Autodesk Inventor part; units mm, degrees
ref_plane "YZ Plane" through (0, 0, 0) normal (1, 0, 0) x (0, 1, 0)
ref_plane "XZ Plane" through (0, 0, 0) normal (0, 1, 0) x (-1, 0, 0)
ref_plane "XY Plane" through (0, 0, 0) normal (0, 0, 1) x (1, 0, 0)
sketch "Boceto1" plane through (0, 0, 0) normal (0, 1, 0) x (-1, 0, 0)
  line L0 (-75, -125) -> (75, -125)
  line L1 (75, -125) -> (75, 125)
  line L2 (75, 125) -> (-75, 125)
  line L3 (-75, 125) -> (-75, -125)
  line L4 (-75, -125) -> (75, 125) construction
  line L5 (75, -125) -> (-75, 125) construction
  line L6 (70, 120) -> (70, -120)
  line L7 (70, -120) -> (-70, -120)
  line L8 (-70, -120) -> (-70, 120)
  line L9 (-70, 120) -> (70, 120)
  line L10 (-75, 125) -> (-75, 100)
  line L11 (-75, 100) -> (-70, 100) construction
  line L12 (-75, 100) -> (-75, 50)
  line L13 (-75, 50) -> (-70, 50) construction
  line L14 (-75, 50) -> (-75, 0)
  line L15 (-75, 100.5) -> (-70, 100.5)
  line L16 (-70, 100.5) -> (-70, 99.5)
  line L17 (-70, 99.5) -> (-75, 99.5)
  line L18 (-75, 99.5) -> (-75, 100.5)
  line L19 (-75, 100.5) -> (-70, 99.5) construction
  line L20 (-70, 100.5) -> (-75, 99.5) construction
  line L21 (-75, 49.5) -> (-70, 49.5)
  line L22 (-70, 49.5) -> (-70, 50.5)
  line L23 (-70, 50.5) -> (-75, 50.5)
  line L24 (-75, 50.5) -> (-75, 49.5)
  line L25 (-75, 49.5) -> (-70, 50.5) construction
  line L26 (-70, 49.5) -> (-75, 50.5) construction
  line L27 (0, 125) -> (-20, 125) construction
  line L28 (-20, 125) -> (-40, 125) construction
  line L29 (-40, 125) -> (-60, 125) construction
  line L30 (-20, 125) -> (-20, 120) construction
  line L31 (-40, 125) -> (-40, 120) construction
  line L32 (-60, 125) -> (-60, 120) construction
  line L33 (-20.5, 120) -> (-19.5, 120)
  line L34 (-19.5, 120) -> (-19.5, 125)
  line L35 (-19.5, 125) -> (-20.5, 125)
  line L36 (-20.5, 125) -> (-20.5, 120)
  line L37 (-20.5, 120) -> (-19.5, 125) construction
  line L38 (-19.5, 120) -> (-20.5, 125) construction
  line L39 (-40.5, 120) -> (-39.5, 120)
  line L40 (-39.5, 120) -> (-39.5, 125)
  line L41 (-39.5, 125) -> (-40.5, 125)
  line L42 (-40.5, 125) -> (-40.5, 120)
  line L43 (-40.5, 120) -> (-39.5, 125) construction
  line L44 (-39.5, 120) -> (-40.5, 125) construction
  line L45 (-60.5, 120) -> (-59.5, 120)
  line L46 (-59.5, 120) -> (-59.5, 125)
  line L47 (-59.5, 125) -> (-60.5, 125)
  line L48 (-60.5, 125) -> (-60.5, 120)
  line L49 (-60.5, 120) -> (-59.5, 125) construction
  line L50 (-59.5, 120) -> (-60.5, 125) construction
  line L51 (0, 125) -> (0, 120) construction
  line L52 (-0.5, 120) -> (0.5, 120)
  line L53 (0.5, 120) -> (0.5, 125)
  line L54 (0.5, 125) -> (-0.5, 125)
  line L55 (-0.5, 125) -> (-0.5, 120)
  line L56 (-0.5, 120) -> (0.5, 125) construction
  line L57 (0.5, 120) -> (-0.5, 125) construction
  line L58 (-70, 0) -> (-75, 0) construction
  line L59 (-75, -0.5) -> (-70, -0.5)
  line L60 (-70, -0.5) -> (-70, 0.5)
  line L61 (-70, 0.5) -> (-75, 0.5)
  line L62 (-75, 0.5) -> (-75, -0.5)
  line L63 (-75, -0.5) -> (-70, 0.5) construction
  line L64 (-70, -0.5) -> (-75, 0.5) construction
  point P0 (0, 0)
  point P1 (-72.5, 100)
  point P2 (-72.5, 50)
  point P3 (-20, 122.5)
  point P4 (-40, 122.5)
  point P5 (-60, 122.5)
  point P6 (0, 122.5)
  point P7 (-72.5, 0)
  point P8 (-75, 0.5)
  point P9 (-75, -0.5)
  point P10 (-70, -0.5)
  point P11 (-75, 50.5)
  point P12 (-75, 49.5)
  point P13 (-70, 100.5)
  point P14 (-0.5, 125)
  point P15 (-0.5, 120)
  point P16 (0.5, 120)
  point P17 (0.5, 125)
  point P18 (-20.5, 125)
  point P19 (-19.5, 125)
  point P20 (-40.5, 125)
  point P21 (-40.5, 120)
  point P22 (-39.5, 120)
  point P23 (-39.5, 125)
  point P24 (-60.5, 120)
  point P25 (-59.5, 120)
  point P26 (-59.5, 125)
  dimension "d0" = 150
  dimension "d1" = 250
  dimension "d2" = 5
  dimension "d5" = 25
  dimension "d6" = 50
  dimension "d7" = 50
  dimension "d8" = 1
  dimension "d9" = 1
  dimension "d10" = 20
  dimension "d11" = 20
  dimension "d12" = 20
  dimension "d13" = 1
  dimension "d14" = 1
  dimension "d15" = 1
  dimension "d16" = 1
  dimension "d17" = 1
extrude "Extrusión1" add sketch "Boceto1" along normal blind 3 contours L3 L59 L8 L7 L6 L9 L53 L2 L1 L0 | L3 L61 L8 L59 | L53 L9 L55 L2 | L3 L21 L8 L61 | L55 L9 L34 L2 | L3 L23 L8 L21 | L34 L9 L36 L2 | L23 L3 L17 L8 | L36 L9 L40 L2 | L17 L3 L15 L8 | L40 L9 L42 L2 | L15 L3 L2 L48 L9 L8 | L42 L9 L46 L2 | L46 L9 L48 L2
extrude "Extrusión2" add sketch "Boceto1" against normal blind 0.2 contours L3 L61 L8 L59 | L53 L9 L55 L2 | L3 L23 L8 L21 | L34 L9 L36 L2 | L17 L3 L15 L8 | L40 L9 L42 L2 | L46 L9 L48 L2
mirror "Simetría1" about plane through (0, 0, 0) normal (1, 0, 0) of "Extrusión2", "Extrusión1"
mirror "Simetría2" about plane through (0, 0, 0) normal (0, 0, 1) of "Extrusión2", "Extrusión1", "Simetría1"
ref_plane "Plano de trabajo1" through (0, 0, 0) normal (1, 0, 0) x (0, 1, 0)
ref_plane "Plano de trabajo2" through (0, 0, 0) normal (-1, 0, 0) x (0, 1, 0)
ref_plane "Plano de trabajo3" through (0, 0, 0) normal (-1, 0, 0) x (0, 1, 0)
properties part number "medidor"
Model file for the job. Use its own axes, mm. A direction names the side the tool comes from. Coordinates: 2 decimals unless noted, no trailing zeros. Loops run counter-clockwise (first coordinate to the right, second up) from the corner with the lowest first, then second, coordinate; pieces in that order, holes last. Notation, with made-up numbers: (67.5, 80.25) - (114.5, 80.25) arc R22 cw to (114.5, 95.25) - close; hole circle Ø5 at (-17.5, -3). An arc over 180 degrees is marked (long way). Write item = value, one per line. Start each with the question number.
Item 1: Saw through at B-B, the plane x = -7.5. List the corners of the cut face in (y, z), then the cut area to 3 significant figures.
Item 2: Saw through at C-C, the plane z = 63. List the corners of the cut face in (x, y), then the cut area to 3 significant figures.
Item 3: Wall check: probe 1 along X at (y, z) = (2.85, 106); probe 2 along Z at (x, y) = (7, 0.45). Give the ranges that are in metal, low to high. Write a range as [from, to].
Item 4: Saw through at A-A, the plane y = 0.6. List the corners of the cut face in (x, z), then the cut area to 3 significant figures.
Item 5: Drop a flat-ended pin along its axis: pin 1 Ø1.5 at (x, z) = (71.5, 64.5) entering from -Y. Give the stop position or say it passes through.
Item 6: 3-axis set-ups, long thin cutter, end or side, ignore diameter. For faces 3 (the face through (73, 0, -75)), 4 (the face through (10, 0, -122)), 5 (the face through (71, 0, 116)): which of +Z, -Z, +X, -X, +Y, -Y reach the whole face in a straight line?
Item 7: Pull direction Z, two halves, no side cores. Call faces 1 (the face through (-71, 0, 116)), 2 (the face through (-72, 0, -25)): +Z half, -Z half, draft (parallel to the pull), parting line (faces both ways), or undercut.
Answers:
q1.outline = (0, -125) - (3, -125) - (3, -120) - (0, -120) - close; (0, 120) - (3, 120) - (3, 125) - (0, 125) - close
q1.area = 30.0 mm2
q2.outline = (-75, 0) - (-70, 0) - (-70, 3) - (-75, 3) - close; (70, 0) - (75, 0) - (75, 3) - (70, 3) - close
q2.area = 30.0 mm2
q3.probe_1 = [-75, -70], [70, 75]
q3.probe_2 = [-125, -120], [120, 125]
q4.outline = (-75, -125) - (75, -125) - (75, 125) - (-75, 125) - close; hole (-70, -120) - (70, -120) - (70, 120) - (-70, 120) - close
q4.area = 3,900 mm2
q5.pin_1 = 0
q6.face_3 = +X, -X, -Y
q6.face_4 = +Z, -Z, -Y
q6.face_5 = +Z, +X, -Y
q7.face_1 = draft
q7.face_2 = undercut
